Check sheet for the modelled part. Datum: model origin and axes. Units: mm. A direction names the side the tool comes from. Coordinates: 2 decimals unless noted, no trailing zeros. Loops run counter-clockwise (first coordinate to the right, second up) from the corner with the lowest first, then second, coordinate; pieces in that order, holes last. Notation, with made-up numbers: (-13, 19.25) - (19, 19.25) arc R37 cw to (19, 58.25) - close; hole circle Ø1 at (30.25, -39). An arc over 180 degrees is marked (long way). Write each question's results on one line, items separated by ' | '. Start each with the question number.
1. Cross-section at D-D (z = 57.15). Record the cut outline in (x, y) (3 decimals), and give its area (3 significant figures).
2. Draft check along Z on faces 1 (the face through (-44.5, 4.7, -44.4)), 2 (the face through (-30.004, 12.501, 3.939)), 3 (the face through (-5.6, 9.525, -18.5)). Enter one of: released by +Z, released by -Z, zero draft, split by the parting line, or undercut.
3. Cross-section at B-B (x = -43.5). Record the cut outline in (y, z) (3 decimals), and give its area (3 significant figures).
4. Gauge pin test, flat ends, axial feed: P1, Ø1.5, axis at x = 40, y = 3.5, coming from the -Z side; P2, Ø7.5, axis at y = 4.5, z = 63, coming from the +X side; P3, Ø10.5, axis at x = -15.5, z = 41.65, coming from the +Y side (3 decimals). Record the tip position at first contact, or that the pin passes through.
5. Cross-section at C-C (y = 6.75). Give the number of separate pieces and of enclosed holes in the cut face, and give its area (3 significant figures).
6. Thickness scan on line 1 (X direction, y = 6.25, z = -32.5); line 2 (Z direction, x = 9, y = 12); line 3 (Z direction, x = -43.5, y = 3). Record the ranges inside material, lowest first. Write a range as [from, to].
7. Tool access check on faces 4 (the face through (14, 4.762, 43)), 5 (the face through (-8.1, 1.41, 9.43)), 6 (the face through (-50.8, 5, 1)). Record the directions out of +Z, -Z, +X, -X, +Y, -Y that give a thin tool (end or side, any length) a straight path to the whole face; none if there is none.
```python
from build123d import *

# Parameters (mm, degrees)
SKETCH4_W                                        = 101.6
SKETCH4_H                                        = 101.6
BOSS_EXTRUDE1_DEPTH                              = 9.525
SKETCH14_R                                       = 26.9875
SKETCH14_R_2                                     = 19.0881
CUT_EXTRUDE2_DEPTH                               = 3.175
MOVE_FACE1_BY                                    = 0.127
MOVE_FACE1_2_BY                                  = 0.127
F_3_8_CLEARANCE_HOLE1_D                          = 13.97
SKETCH19_W                                       = 43.7
SKETCH19_H                                       = 28.2
BOSS_EXTRUDE4_DEPTH                              = 9.525
CBORE_FOR_M3_SHCS1_D                             = 3.4
CBORE_FOR_M3_SHCS1_CBORE_D                       = 6.5
CBORE_FOR_M3_SHCS1_CBORE_DEPTH                   = 3
MOVE_FACE4_BY                                    = 1.5875
MOVE_FACE4_2_BY                                  = 1.5875
MOVE_FACE4_3_BY                                  = 1.5875
MOVE_FACE4_4_BY                                  = 1.5875
SKETCH11_R                                       = 12.7
CUT_EXTRUDE1_DEPTH                               = 95.405326253
CHAMFER1_SIZE                                    = 0.79375
BODY_MOVE_COPY2_ANGLE                            = 180
SKETCH21_R                                       = 3.25
CUT_EXTRUDE3_DEPTH                               = 4.7625
CHAMFER2_SIZE                                    = 12.7
CHAMFER3_SIZE                                    = 6.35
CBORE_FOR_1_4_SOCKET_HEAD_CAP_SCREW1_D           = 6.7564
CBORE_FOR_1_4_SOCKET_HEAD_CAP_SCREW1_CBORE_D     = 11.1125
CBORE_FOR_1_4_SOCKET_HEAD_CAP_SCREW1_CBORE_DEPTH = 6.35
MIRROR2_COPY_1_D                                 = 6.7564
MIRROR2_COPY_1_CBORE_D                           = 11.1125
MIRROR2_COPY_1_CBORE_DEPTH                       = 6.35


with BuildPart() as part:
    # Sketch4 → Boss-Extrude1 (new body)
    with BuildSketch(Plane(origin=(0, 0, 0), x_dir=(1, 0, 0), z_dir=(0, 1, 0))):
        Rectangle(SKETCH4_W, SKETCH4_H)
    extrude(amount=BOSS_EXTRUDE1_DEPTH)

    # Sketch5 → Revolve1 (revolve)
    with BuildSketch(Plane(origin=(0, 0, 0), x_dir=(0, 0, -1), z_dir=(1, 0, 0))):
        Polygon((0, 9.525), (0, 12.7), (30.1625, 12.7), (31.75, 9.525), align=None)
    revolve(axis=Axis((0, 0, 0), (0, 1, 0)))

    # Sketch14 → Cut-Extrude2 (cut)
    with BuildSketch(Plane(origin=(0, 12.7, 0), x_dir=(1, 0, 0), z_dir=(0, 1, 0))):
        with Locations(Location((0, 0, 0), (0, 0, 270))):
            Circle(SKETCH14_R)
        with Locations(Location((0, 0, 0), (0, 0, 270))):
            Circle(SKETCH14_R_2, mode=Mode.SUBTRACT)
    extrude(amount=-CUT_EXTRUDE2_DEPTH, mode=Mode.SUBTRACT)

    # Move Face1: a curved face moved inward by 0.127
    add(Solid.thicken(part.faces().sort_by_distance((0, 11.1125, -19.0881))[0], -MOVE_FACE1_BY), mode=Mode.SUBTRACT)

    # Move Face1 2: a curved face moved inward by 0.127
    add(Solid.thicken(part.faces().sort_by_distance((0, 11.1125, -26.9875))[0], -MOVE_FACE1_2_BY), mode=Mode.SUBTRACT)

    # 3/8 Clearance Hole1 (through all)
    with Locations(Plane(origin=(0, 12.7, 0), x_dir=(1, 0, 0), z_dir=(0, 1, 0))):
        with Locations((0, 0)):
            Hole(F_3_8_CLEARANCE_HOLE1_D / 2)

    # Sketch19 → Boss-Extrude4 (add)
    with BuildSketch(Plane(origin=(0, 9.525, 0), x_dir=(1, 0, 0), z_dir=(0, 1, 0))):
        with Locations((0, -64.9)):
            Rectangle(SKETCH19_W, SKETCH19_H)
    extrude(amount=-BOSS_EXTRUDE4_DEPTH)

    # CBORE for M3 SHCS1 (through all)
    with Locations(Plane(origin=(0, 9.525, 0), x_dir=(1, 0, 0), z_dir=(0, 1, 0))):
        with Locations((-15.5, -41.65), (15.5, -41.65), (15.5, -72.65), (-15.5, -72.65)):
            CounterBoreHole(CBORE_FOR_M3_SHCS1_D / 2, CBORE_FOR_M3_SHCS1_CBORE_D / 2, CBORE_FOR_M3_SHCS1_CBORE_DEPTH)

    # Move Face4: a face moved inward by 1.5875
    extrude(part.faces().sort_by_distance((15.5, 6.525, 44.25))[0], amount=MOVE_FACE4_BY, dir=(0, -1, 0), mode=Mode.SUBTRACT)

    # Move Face4 2: a face moved inward by 1.5875
    extrude(part.faces().sort_by_distance((-15.5, 6.525, 44.25))[0], amount=MOVE_FACE4_2_BY, dir=(0, -1, 0), mode=Mode.SUBTRACT)

    # Move Face4 3: a face moved inward by 1.5875
    extrude(part.faces().sort_by_distance((-15.5, 6.525, 75.25))[0], amount=MOVE_FACE4_3_BY, dir=(0, -1, 0), mode=Mode.SUBTRACT)

    # Move Face4 4: a face moved inward by 1.5875
    extrude(part.faces().sort_by_distance((15.5, 6.525, 75.25))[0], amount=MOVE_FACE4_4_BY, dir=(0, -1, 0), mode=Mode.SUBTRACT)

    # Sketch11 → Cut-Extrude1 (cut, through all)
    with BuildSketch(Plane(origin=(0, 9.525, 0), x_dir=(1, 0, 0), z_dir=(0, 1, 0))):
        with Locations(Location((0, -57.15, 0), (0, 0, 270))):
            Circle(SKETCH11_R)
    extrude(amount=-CUT_EXTRUDE1_DEPTH, mode=Mode.SUBTRACT)

    # Chamfer1
    chamfer1_edges = [part.edges().sort_by_distance(p)[0] for p in [
        (0, 12.7, -27.1145),
        (0, 12.7, -18.9611),
    ]]
    chamfer(chamfer1_edges, length=CHAMFER1_SIZE)


with BuildPart() as body_2:
    # uxcell-FR6ZZ: read off the stored shape, not the designer's step
    # uxcell-FR6ZZ outline → uxcell-FR6ZZ (revolve)
    with BuildSketch(Plane(origin=(-24.054896115, 0, 40.177492641), x_dir=(1, 0, 0), z_dir=(0, 0, 1))):
        Polygon((12.430125, -6.322384388), (4.7625, -6.322384388), (4.7625, -14.736134388), (11.2395, -14.736134388), (11.2395, -9.576759388), (11.636375, -9.179884388), (12.430125, -9.179884388), align=None)
    revolve(axis=Axis((-24.054896115, 0, 40.177492641), (0, 1, 0)))


with BuildPart() as body_2_1:
    # Body-Move/Copy2: read off the stored shape, not the designer's step
    # Body-Move/Copy2: moved
    add(body_2.part.moved(Location((24.0548961, 6.3223844, -40.1774926))).rotate(Axis((0, 0, 0), (0.9584281675, 0, 0.2853339234)), BODY_MOVE_COPY2_ANGLE))


with BuildPart() as part_1:
    add(part.part)

    # Combine1: cut body 2
    add(body_2_1.part, mode=Mode.SUBTRACT)

    # Sketch21 → Cut-Extrude3 (cut)
    with BuildSketch(Plane(origin=(0, 9.525, 0), x_dir=(1, 0, 0), z_dir=(0, 1, 0))):
        with Locations(Location((-15.5, -72.65, 0), (0, 0, 270))):
            Circle(SKETCH21_R)
        with Locations(Location((15.5, -72.65, 0), (0, 0, 270))):
            Circle(SKETCH21_R)
        with Locations(Location((15.5, -41.65, 0), (0, 0, 270))):
            Circle(SKETCH21_R)
        with Locations(Location((-15.5, -41.65, 0), (0, 0, 270))):
            Circle(SKETCH21_R)
    extrude(amount=-CUT_EXTRUDE3_DEPTH, mode=Mode.SUBTRACT)

    # Chamfer2
    chamfer2_edges = [part_1.edges().sort_by_distance(p)[0] for p in [
        (50.8, 4.7625, 50.8),
        (-50.8, 4.7625, 50.8),
        (-50.8, 4.7625, -50.8),
        (50.8, 4.7625, -50.8),
    ]]
    chamfer(chamfer2_edges, length=CHAMFER2_SIZE)

    # Chamfer3
    chamfer3_edges = [part_1.edges().sort_by_distance(p)[0] for p in [
        (-21.85, 4.7625, 79),
        (21.85, 4.7625, 79),
    ]]
    chamfer(chamfer3_edges, length=CHAMFER3_SIZE)

    # CBORE for 1/4 Socket Head Cap Screw1 (through all)
    with Locations(Plane(origin=(0, 9.525, 0), x_dir=(1, 0, 0), z_dir=(0, 1, 0))):
        with Locations((-44.500451365, 32.095919635), (-44.500451365, 22.570919635)):
            cbore_for_1_4_socket_head_cap_screw1 = CounterBoreHole(CBORE_FOR_1_4_SOCKET_HEAD_CAP_SCREW1_D / 2, CBORE_FOR_1_4_SOCKET_HEAD_CAP_SCREW1_CBORE_D / 2, CBORE_FOR_1_4_SOCKET_HEAD_CAP_SCREW1_CBORE_DEPTH)

    # Mirror1: CBORE for 1/4 Socket Head Cap Screw1 across plane
    add(cbore_for_1_4_socket_head_cap_screw1.mirror(Plane.XY), mode=Mode.SUBTRACT)

    # Mirror2: CBORE for 1/4 Socket Head Cap Screw1 across plane
    add(cbore_for_1_4_socket_head_cap_screw1.mirror(Plane(origin=(0, 0, 0), x_dir=(0, 0, 1), z_dir=(1, 0, 0))), mode=Mode.SUBTRACT)

    # Mirror2 copy 1 (through all)
    with Locations(Plane(origin=(0, 9.525, 0), x_dir=(-1, 0, 0), z_dir=(0, 1, 0))):
        with Locations((-44.500451365, 32.095919635), (-44.500451365, 22.570919635)):
            CounterBoreHole(MIRROR2_COPY_1_D / 2, MIRROR2_COPY_1_CBORE_D / 2, MIRROR2_COPY_1_CBORE_DEPTH)


solid = part_1.part
```
Established:
1) outline: (-21.85, 0) - (-12.7, 0) - (-12.7, 9.525) - (-21.85, 9.525) - close; (12.7, 0) - (21.85, 0) - (21.85, 9.525) - (12.7, 9.525) - close | area: 174 mm^2
2) face 1: released by -Z | face 2: split by the parting line | face 3: undercut
3) outline: (0, -45.4) - (9.525, -45.4) - (9.525, -37.561) - (3.175, -37.561) - (3.175, -35.323) - (0, -35.323) - close; (0, -28.869) - (3.175, -28.869) - (3.175, -25.798) - (0, -25.798) - close; (0, -19.344) - (3.175, -19.344) - (3.175, -17.105) - (9.525, -17.105) - (9.525, 17.105) - (3.175, 17.105) - (3.175, 19.344) - (0, 19.344) - close; (0, 25.798) - (3.175, 25.798) - (3.175, 28.869) - (0, 28.869) - close; (0, 35.323) - (3.175, 35.323) - (3.175, 37.561) - (9.525, 37.561) - (9.525, 45.4) - (0, 45.4) - close | area: 523 mm^2
4) P1: z = -49.65 | P2: x = 21.85 | P3: y = 9.525
5) separate pieces: 1 | enclosed holes: 10 | area: 9,400 mm^2
6) line 1: [-50.8, -50.04], [-38.96, 38.96], [50.04, 50.8] | line 2: [-29.15, -25.68], [-16.58, 16.58], [25.68, 29.15] | line 3: [-45.4, -35.32], [-28.87, -25.8], [-19.34, 19.34], [25.8, 28.87], [35.32, 45.4]
7) face 4: +Y | face 5: -Y | face 6: +Z, -Z, -X, +Y, -Y
